For this review, take the finished solid that the model builds, in its own axes (mm). Face numbers are marked on the shaded views. A direction names the side the tool comes from. Give positions to 0.01 mm unless a question says otherwise; leave off trailing zeros. Order: outer loops, then holes, each group sorted by start corner. A loop starts at its lowest first (then second) coordinate and runs counter-clockwise, first axis right, second up.
from build123d import *

# Parameters (mm, degrees)
F6_DEPTH        = 21
F7_SIZE         = 2
F8_SIZE         = 2
F12_DEPTH       = 2.5510001
F14_D           = 2.5
F14_CSINK_D     = 4
F14_CSINK_ANGLE = 90


# Not quite as in the source:
# - a feature names something its author has since deleted; it is built from what else it names


with BuildPart() as f6:
    # F5 (on Front) → F6 (new body)
    with BuildSketch(Plane.XZ):
        with BuildLine():
            ThreePointArc((1.75, 9.3374246985), (3.2970633562, 8.9095102685), (4.75, 8.227241336))
            Line((4.75, 8.227241336), (4.75, 13.027241336))
            Line((4.75, 13.027241336), (-4.75, 13.027241336))
            Line((-4.75, 13.027241336), (-4.75, 8.227241336))
            ThreePointArc((-4.75, 8.227241336), (-3.2970633562, 8.9095102685), (-1.75, 9.3374246985))
            Line((-1.75, 9.3374246985), (-1.75, 10.777241336))
            ThreePointArc((-1.75, 10.777241336), (0, 12.527241336), (1.75, 10.777241336))
            Line((1.75, 10.777241336), (1.75, 9.3374246985))
        make_face()
        with BuildLine():
            ThreePointArc((-1.75, 9.3374246985), (0, 9.5), (1.75, 9.3374246985))
            Line((1.75, 9.3374246985), (1.75, 10.777241336))
            ThreePointArc((1.75, 10.777241336), (0, 12.527241336), (-1.75, 10.777241336))
            Line((-1.75, 10.777241336), (-1.75, 9.3374246985))
        make_face()
    extrude(amount=-F6_DEPTH)

    # F7
    f7_edges = [f6.edges().sort_by_distance(p)[0] for p in [
        (-4.75, 10.5, 13.027241),
        (4.75, 10.5, 13.027241),
    ]]
    chamfer(f7_edges, length=F7_SIZE)

    # F8
    f8_edges = [f6.edges().sort_by_distance(p)[0] for p in [
        (0, 21, 13.027241),
    ]]
    chamfer(f8_edges, length=F8_SIZE)

    # F10 (on offset) → F11 (revolve, cut)
    with BuildSketch(Plane.XY.offset(10.777241336)):
        with BuildLine():
            Line((-1.75, 11.75), (-1.75, 0))
            Line((-1.75, 0), (0, 0))
            Line((0, 0), (0, 13.5))
            ThreePointArc((0, 13.5), (-1.2374368671, 12.9874368671), (-1.75, 11.75))
        make_face()
    revolve(axis=Axis((0, 6.75, 10.777241336), (0, 1, 0)), mode=Mode.SUBTRACT)

    # F10 (on offset) → F12 (cut, through all)
    with BuildSketch(Plane.XY.offset(10.777241336)):
        with BuildLine():
            Line((0, 13.5), (0, 0))
            Line((0, 0), (1.75, 0))
            Line((1.75, 0), (1.75, 11.75))
            ThreePointArc((1.75, 11.75), (1.2374368671, 12.9874368671), (0, 13.5))
        make_face()
        with BuildLine():
            Line((-1.75, 11.75), (-1.75, 0))
            Line((-1.75, 0), (0, 0))
            Line((0, 0), (0, 13.5))
            ThreePointArc((0, 13.5), (-1.2374368671, 12.9874368671), (-1.75, 11.75))
        make_face()
    extrude(amount=-F12_DEPTH, mode=Mode.SUBTRACT)

    # F14 (through all)
    with Locations(Plane.XY.offset(13.027241336)):
        with Locations((0, 16)):
            CounterSinkHole(F14_D / 2, F14_CSINK_D / 2, counter_sink_angle=F14_CSINK_ANGLE)


solid = f6.part
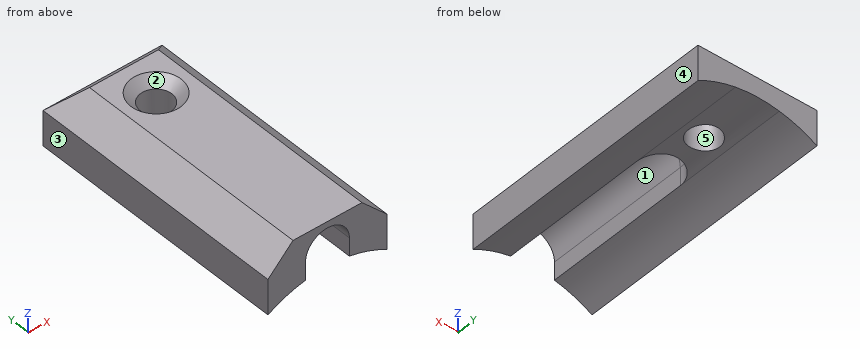
1) We need section C-C on y = 2.75. Give the boundary of the cut face in (x, z).
Answer sheet:
outline: (-4.75, 8.23) arc R9.5 cw to (-1.75, 9.34) - (-1.75, 10.78) arc R1.75 cw to (1.75, 10.78) - (1.75, 9.34) arc R9.5 cw to (4.75, 8.23) - (4.75, 11.03) - (2.75, 13.03) - (-2.75, 13.03) - (-4.75, 11.03) - close
2) We need section A-A on y = 16. Give the boundary of the cut face in (x, z), then the cut area to 3 significant figures.
Answer sheet:
outline: (-4.75, 8.23) arc R9.5 cw to (-1.25, 9.42) - (-1.25, 12.28) - (-2, 13.03) - (-2.75, 13.03) - (-4.75, 11.03) - close; (1.25, 9.42) arc R9.5 cw to (4.75, 8.23) - (4.75, 11.03) - (2.75, 13.03) - (2, 13.03) - (1.25, 12.28) - close
area: 24.0 mm2
3) Draft analysis for pull direction X (two halves, no side actions). For the marked faces 3, 4 and 5, state which applies: +X half, -X half, draft (parallel to the pull), parting line (faces both ways), or undercut.
Answer sheet:
face 3: -X half
face 4: +X half
face 5: undercut
4) We need section B-B on z = 10. Give the boundary of the cut face in (x, y).
Answer sheet:
outline: (-4.75, 0) - (-1.75, 0) - (-1.75, 11.75) arc R1.75 cw to (1.75, 11.75) - (1.75, 0) - (4.75, 0) - (4.75, 21) - (-4.75, 21) - close; hole circle Ø2.5 at (0, 16)
5) We need section D-D on x = 4. Give the boundary of the cut face in (y, z).
Answer sheet:
outline: (0, 8.62) - (21, 8.62) - (21, 11.03) - (20.25, 11.78) - (0, 11.78) - close
6) To check wall thickness, follow line 1 (Y direction, x = 0, z = 10.3); line 2 (X direction, y = 16, z = 10.5); line 3 (X direction, y = 15, z = 8.5). State the ranges of each line that lie inside material, in increasing order.
Answer sheet:
line 1: y = 13.5 to 14.75, 17.25 to 21
line 2: x = -4.75 to -1.25, 1.25 to 4.75
line 3: x = -4.75 to -4.24, 4.24 to 4.75
7) Tool access review of the marked faces 1 and 2: name each direction out of +Z, -Z, +X, -X, +Y, -Y from which nothing blocks a thin tool from reaching the whole face with its end or side.
Answer sheet:
face 1: -Z, -Y
face 2: +Z
8) Clearance check with flat-ended pins moving along their axes: pin 1 (3 mm diameter, centred on x = 0, y = 16, fed in from +Z); pin 2 (3 mm diameter, centred on x = 1, y = 5, fed in from -Z). State where each tip first meets the part, or that it passes through.
Answer sheet:
pin 1: stops at z = 12.53
pin 2: stops at z = 9.17
